The model under review builds one solid part; all positions refer to its coordinate system, in mm. Give positions to 0.01 mm unless a question says otherwise; leave off trailing zeros. Order: outer loops, then holes, each group sorted by start corner. A loop starts at its lowest first (then second) coordinate and runs counter-clockwise, first axis right, second up. Notation, with made-up numbers: M -34.5,-11 L -0.5,-11 A8 cw -0.5,2 Z; hole C -36,-21 d2. An arc over 180 degrees is marked long. One line per question, with ' | ' between items. Start each with the question number.
1. Wall thickness on L1, parallel to X at y = 1.8, z = 0; L2, parallel to Z at x = 1, y = 2; L3, parallel to X at y = 2.2, z = 1.5: over which ranges is each line inside the solid? List them lowest first.
2. We need section D-D on y = 2.7. Write out the cut boundary in (x, z).
3. Insertion check: P1, Ø1.5, axis at x = 1, y = 2, coming from the +Z side; P2, Ø1.5, axis at y = 0.5, z = -3, coming from the +X side; P3, Ø1.5, axis at x = 1.5, y = 1.5, coming from the -Z side; P4, Ø1, axis at x = 1.5, z = 3, coming from the +Y side. Each pin has a flat end and moves straight along its axis. Give the tip position at first contact, or say it passes through.
4. We need section C-C on y = 0.85. Write out the cut boundary in (x, z).
5. We need section B-B on z = 0. Write out the cut boundary in (x, y), then the cut area to 3 significant figures.
6. The part is to be moulded in two halves that separate along Z. For faces 1 (the face through (-1, 1.48, -1.31)), 2 (the face through (-1.4, 3, 1.4)), 3 (the face through (-2.343, 1.485, -3.055)), say which applies: +Z half, -Z half, draft (parallel to the pull), parting line (faces both ways), or undercut.
7. We need section A-A on x = 0. Write out the cut boundary in (y, z), then the cut area to 3 significant figures.
```python
from build123d import *

# Parameters (mm, degrees)
SKETCH_1_R       = 3.85
SKETCH_1_R_2     = 1.65
EXTRUDE_1_DEPTH  = 3
CHAMFER_8_SIZE   = 0.4
CHAMFER_8_SIZE2  = 0.692820323
CHAMFER_10_SIZE  = 0.4
CHAMFER_10_SIZE2 = 0.692820323


with BuildPart() as part:
    # Эскиз1 → Бобышка-Вытянуть1 (new body)
    with BuildSketch(Plane(origin=(0, 0, 0), x_dir=(1, 0, 0), z_dir=(0, 1, 0))):
        with Locations(Location((0, 0, 0), (0, 0, 270))):
            Circle(SKETCH_1_R)
        with Locations(Location((0, 0, 0), (0, 0, 270))):
            Circle(SKETCH_1_R_2, mode=Mode.SUBTRACT)
    extrude(amount=EXTRUDE_1_DEPTH)

    # Фаска8
    chamfer_8_edges = [part.edges().sort_by_distance(p)[0] for p in [
        (0, 3, -3.85),
    ]]
    chamfer_8_side = [part.faces().sort_by_distance(p)[0] for p in [
        (0, 1.5, -3.85),
    ]]
    chamfer(chamfer_8_edges, length=CHAMFER_8_SIZE, length2=CHAMFER_8_SIZE2, reference=chamfer_8_side[0])

    # Фаска10
    chamfer_10_edges = [part.edges().sort_by_distance(p)[0] for p in [
        (0, 0, -3.85),
    ]]
    chamfer_10_side = [part.faces().sort_by_distance(p)[0] for p in [
        (0, 1.3, -3.85),
    ]]
    chamfer(chamfer_10_edges, length=CHAMFER_10_SIZE, length2=CHAMFER_10_SIZE2, reference=chamfer_10_side[0])


solid = part.part
```
Entries:
1) L1: x = -3.85 to -1.65, 1.65 to 3.85 | L2: z = -3.72 to -1.31, 1.31 to 3.72 | L3: x = -3.55 to -0.69, 0.69 to 3.55
2) outline: C 0,0 d7.35; hole C 0,0 d3.3
3) P1: stops at z = 3.84 | P2: stops at x = 3.12 | P3: stops at z = -3.78 | P4: stops at y = 3
4) outline: C 0,0 d7.7; hole C 0,0 d3.3
5) outline: M -3.85,0.4 L -3.16,0 L -1.65,0 L -1.65,3 L -3.16,3 L -3.85,2.6 Z; M 1.65,0 L 3.16,0 L 3.85,0.4 L 3.85,2.6 L 3.16,3 L 1.65,3 Z | area: 12.6 mm^2
6) face 1: undercut | face 2: draft | face 3: parting line
7) outline: M 0,-3.16 L 0.4,-3.85 L 2.6,-3.85 L 3,-3.16 L 3,-1.65 L 0,-1.65 Z; M 0,1.65 L 3,1.65 L 3,3.16 L 2.6,3.85 L 0.4,3.85 L 0,3.16 Z | area: 12.6 mm^2
